Geometry check sheet. Reference: the model listing, model coordinates, mm. Face numbers are marked on the shaded views. A direction names the side the tool comes from. Coordinates: 2 decimals unless noted, no trailing zeros. Loops run counter-clockwise (first coordinate to the right, second up) from the corner with the lowest first, then second, coordinate; pieces in that order, holes last. Notation, with made-up numbers: (23, 36) - (58, 36) arc R25 cw to (58, 66) - close; hole circle Ø1 at (-9.75, 17). An arc over 180 degrees is marked (long way). Write item = value, one per line. Start each with the question number.
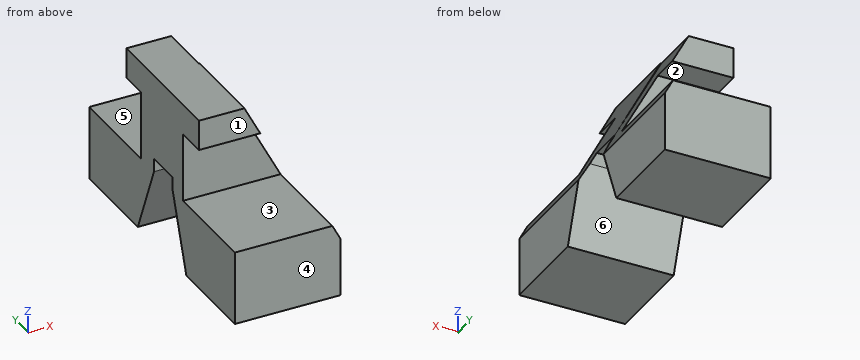
from build123d import *

# Parameters (mm, degrees)
F1_DEPTH = 43.434
F3_DEPTH = 57.404
F5_DEPTH = 71.628


with BuildPart() as f1:
    # F0 (on Right) → F1 (new body)
    with BuildSketch(Plane.YZ):
        Polygon((21.547339, 40.943282), (-35.326082, 40.943282), (-35.326082, 28.432836), (-22.815635, 28.432836), (-22.86, 0), (-63.5, 0), (-63.5, -30.48), (-25.4, -30.48), (-14.66608, 0), (-14.66608, 5.442686), (0, 5.442686), (0, 0), (12.7, -30.48), (50.8, -30.48), (50.8, 0), (10.16, 0), (10.16, 28.311027), (21.547339, 28.311027), align=None)
    extrude(amount=F1_DEPTH)

    # F2 (on Front) → F3 (cut)
    with BuildSketch(Plane.XZ):
        Polygon((15.067352, 47.276348), (45.27159, -9.890955), (45.27159, 47.276348), align=None)
    extrude(amount=-F3_DEPTH, mode=Mode.SUBTRACT)

    # F4 (on Front) → F5 (cut)
    with BuildSketch(Plane.XZ):
        Polygon((17.860672, 42.400945), (45.15991, -9.874192), (45.15991, 42.400945), align=None)
    extrude(amount=F5_DEPTH, mode=Mode.SUBTRACT)


solid = f1.part
(1) Sectioned sample at C-C on x = 7. Enter the section's corners in (y, z).
(2) Tool access check on the marked faces 1, 2 and 3. Record the directions out of +Z, -Z, +X, -X, +Y, -Y that give a thin tool (end or side, any length) a straight path to the whole face; none if there is none.
(3) Depth check by flat-ended pin: pin 1 (9 mm diameter, centred on x = 25.5, z = 25.5, fed in from +Y); pin 2 (2.5 mm diameter, centred on x = 19, z = 2, fed in from +Y); pin 3 (4 mm diameter, centred on x = 12.5, z = 37, fed in from -Y). Enter the tip coordinate at first touch or a pass-through.
(4) Sectioned sample at A-A on y = 11.5. Enter the section's corners in (x, z).
(5) Draft check along Y on the marked faces 4, 5 and 6. Enter one of: pulls with the +Y half, pulls with the -Y half, needs draft (parallel to the pull), parting line crosses it, or undercut.
(6) Sectioned sample at B-B on z = 2. Enter the section's corners in (x, y), plus the area to 3 significant figures.
(7) Sectioned sample at D-D on y = -29.5. Enter the section's corners in (x, z).
(8) Scan lines: line 1 (Z direction, x = 3, y = 13.5); line 2 (Y direction, x = 14.5, z = 9); line 3 (Y direction, x = 17.5, z = 33). Record each from-to range of solid material in increasing order.
Working result:
q1.outline = (-63.5, -30.48) - (-25.4, -30.48) - (-14.67, 0) - (-14.67, 5.44) - (0, 5.44) - (0, 0) - (12.7, -30.48) - (50.8, -30.48) - (50.8, 0) - (10.16, 0) - (10.16, 28.31) - (21.55, 28.31) - (21.55, 40.94) - (-35.33, 40.94) - (-35.33, 28.43) - (-22.82, 28.43) - (-22.86, 0) - (-63.5, 0) - close
q2.face_1 = +Z, +X, -X, -Y
q2.face_2 = +X, -X, +Y
q2.face_3 = +X, -X, -Y
q3.pin_1 = 21.55
q3.pin_2 = 10.16
q3.pin_3 = -35.33
q4.outline = (0, -27.6) - (43.43, -27.6) - (43.43, -6.41) - (40.05, 0) - (0, 0) - close; (0, 28.31) - (25.09, 28.31) - (18.41, 40.94) - (0, 40.94) - close
q5.face_4 = pulls with the -Y half
q5.face_5 = needs draft
q5.face_6 = undercut
q6.outline = (0, -22.86) - (38.96, -22.86) - (38.96, -14.67) - (0, -14.67) - close; (0, 0) - (38.99, 0) - (38.99, 10.16) - (0, 10.16) - close
q6.area = 715 mm2
q7.outline = (0, -30.48) - (43.43, -30.48) - (43.43, -6.57) - (40, 0) - (0, 0) - close; (0, 28.43) - (25.16, 28.43) - (18.62, 40.94) - (0, 40.94) - close
q8.line_1 = -30.48 to 0, 28.31 to 40.94
q8.line_2 = -22.85 to 10.16
q8.line_3 = -35.33 to 21.55
